```python
from build123d import *

# Parameters (mm, degrees)
CROQUIS1_R              = 2.75
SALIENTE_EXTRUIR1_DEPTH = 1
CROQUIS2_R              = 2.45
SALIENTE_EXTRUIR2_DEPTH = 5.05
C_PULA1_FACE_RADIUS     = 2.45
C_PULA1_HEIGHT          = 2.45
CROQUIS3_R              = 0.25
SALIENTE_EXTRUIR3_DEPTH = 16
CROQUIS5_R              = 0.25
SALIENTE_EXTRUIR5_DEPTH = 17


with BuildPart() as part:
    # Croquis1 → Saliente-Extruir1 (new body)
    with BuildSketch(Plane(origin=(0, 0, 0), x_dir=(1, 0, 0), z_dir=(0, 1, 0))):
        with Locations(Location((0, 0, 0), (0, 0, 270))):
            Circle(CROQUIS1_R)
    extrude(amount=SALIENTE_EXTRUIR1_DEPTH)

    # Croquis2 → Saliente-Extruir2 (add)
    with BuildSketch(Plane(origin=(0, 1, 0), x_dir=(1, 0, 0), z_dir=(0, 1, 0))):
        with Locations(Location((0, 0, 0), (0, 0, 270))):
            Circle(CROQUIS2_R)
    extrude(amount=SALIENTE_EXTRUIR2_DEPTH)

    # Cúpula1: a dome of height H over a round flat face of radius A is a cap of a sphere of radius (A * A + H * H) / (2 * H)
    c_pula1_r = (C_PULA1_FACE_RADIUS * C_PULA1_FACE_RADIUS + C_PULA1_HEIGHT * C_PULA1_HEIGHT) / (2 * C_PULA1_HEIGHT)
    c_pula1_base = Plane((0, 6.05, 0), z_dir=(0, 1, 0))
    with Locations(c_pula1_base.offset(C_PULA1_HEIGHT - c_pula1_r)):
        c_pula1_ball = Sphere(c_pula1_r, mode=Mode.PRIVATE)
    add(split(c_pula1_ball, bisect_by=c_pula1_base, keep=Keep.TOP, mode=Mode.PRIVATE))

    # Croquis3 → Saliente-Extruir3 (add)
    with BuildSketch(Plane.XZ):
        with Locations(Location((-1.205162028, 0, 0), (0, 0, 90))):
            Circle(CROQUIS3_R)
    extrude(amount=SALIENTE_EXTRUIR3_DEPTH)

    # Croquis5 → Saliente-Extruir5 (add)
    with BuildSketch(Plane.XZ):
        with Locations(Location((1.205162028, 0, 0), (0, 0, 90))):
            Circle(CROQUIS5_R)
    extrude(amount=SALIENTE_EXTRUIR5_DEPTH)


solid = part.part
```
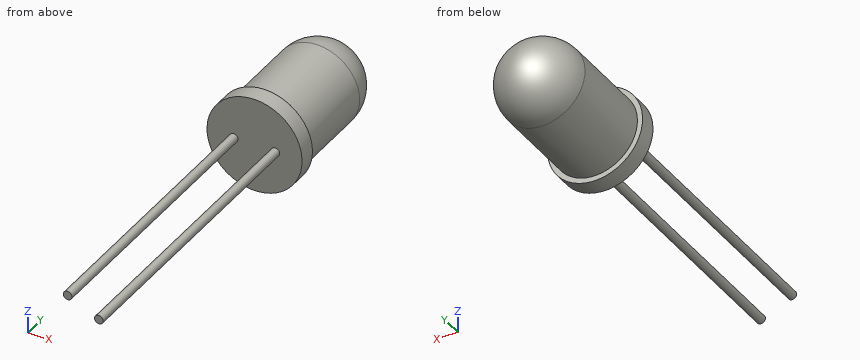
Work out the finished part from the listing and answer in its coordinate system (mm). Give positions to 0.01 mm unless a question says otherwise; leave off trailing zeros. Loops run counter-clockwise (first coordinate to the right, second up) from the corner with the lowest first, then second, coordinate; pieces in that order, holes last. Notation, with made-up numbers: (-35, 26.25) -> (23, 26.25) arc R13 ccw to (23, 36.25) -> close; hole circle Ø8 at (79.5, -26.5). An arc over 180 degrees is marked (long way). Write item = value, one per line. Start each with the question number.
(1) Find section A-A on x = 0. Give the vertices of the cut face in (y, z).
(2) Find section B-B on z = 0. Give the vertices of the cut face in (x, y), and give its area (3 significant figures).
(3) Find section C-C on y = 4. Give the vertices of the cut face in (x, z).
(4) Find the intervals of material crossed by probe 1 along X at (y, z) = (-11.75, 0.05); probe 2 along Z at (x, y) = (-0.15, 2.5); probe 3 along X at (y, z) = (-11.25, -0.15), in increasing order. Write a range as from..to.
(5) Find section D-D on x = -2.05. Give the vertices of the cut face in (y, z), and give its area (3 significant figures).
(6) Given pin 1 Ø1 at (x, z) = (0.5, 1.5) entering from -Y; pin 2 Ø1.6 at (x, z) = (-1, -1) entering from +Y; pin 3 Ø1.5 at (x, z) = (1, 1.5) entering from +Y, each flat-ended and moving along its own axis, determine where each tip first touches the part or whether it passes through.
From the geometry:
q1.outline = (0, -2.75) -> (1, -2.75) -> (1, -2.45) -> (6.05, -2.45) arc R2.45 ccw to (6.05, 2.45) -> (1, 2.45) -> (1, 2.75) -> (0, 2.75) -> close
q2.outline = (-2.75, 0) -> (-1.46, 0) -> (-1.46, -16) -> (-0.96, -16) -> (-0.96, 0) -> (0.96, 0) -> (0.96, -17) -> (1.46, -17) -> (1.46, 0) -> (2.75, 0) -> (2.75, 1) -> (2.45, 1) -> (2.45, 6.05) arc R2.45 ccw to (-2.45, 6.05) -> (-2.45, 1) -> (-2.75, 1) -> close
q2.area = 56.2 mm^2
q3.outline = circle Ø4.9 at (0, 0)
q4.probe_1 = -1.45..-0.96, 0.96..1.45
q4.probe_2 = -2.45..2.45
q4.probe_3 = -1.41..-1.01, 1.01..1.41
q5.outline = (0, -1.83) -> (1, -1.83) -> (1, -1.34) -> (6.05, -1.34) arc R1.34 ccw to (6.05, 1.34) -> (1, 1.34) -> (1, 1.83) -> (0, 1.83) -> close
q5.area = 20.0 mm^2
q6.pin_1 = 0
q6.pin_2 = 8.42
q6.pin_3 = 8.26
